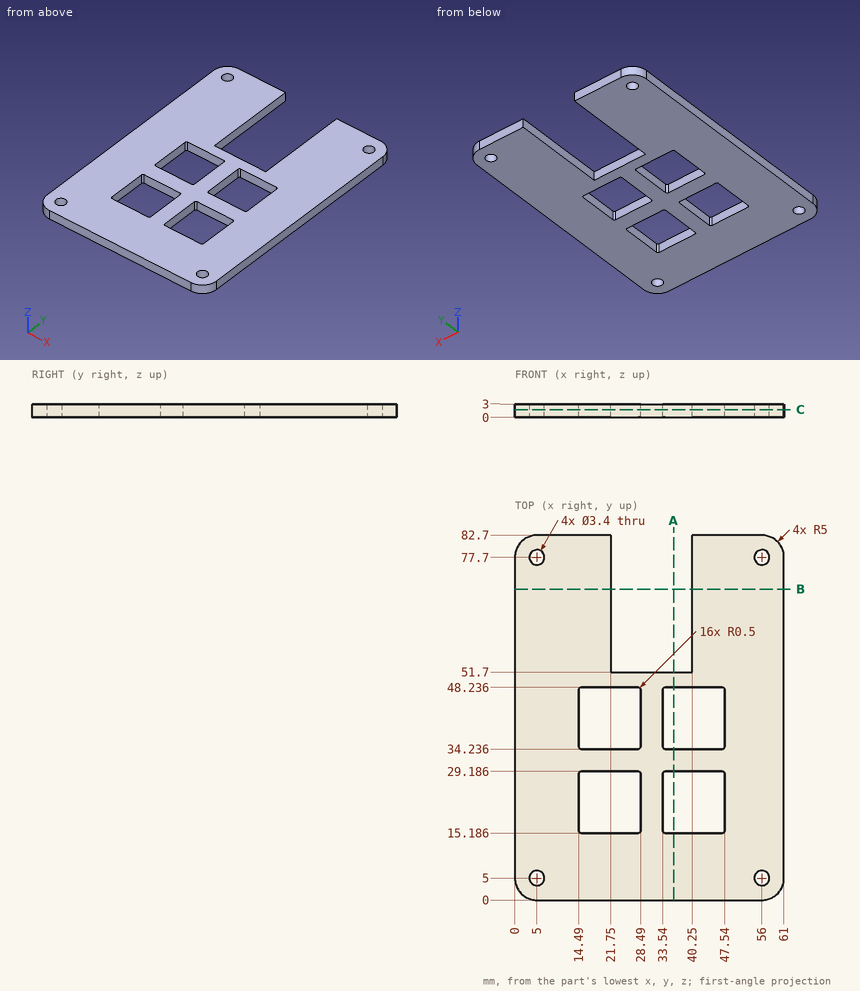
Check sheet for the drawn part. Datum: minimum x, y, z corner. Units: mm. Round coordinates to 2 decimals unless told otherwise and drop trailing zeros. Loops run counter-clockwise (first coordinate to the right, second up) from the corner with the lowest first, then second, coordinate; pieces in that order, holes last. Notation, with made-up numbers: (-37.75, 28.25) - (12.25, 28.25) arc R8 ccw to (12.25, 36.25) - close; hole circle Ø1 at (83.25, -3.75). An arc over 180 degrees is marked (long way). Answer as a JSON object with one key per item and string values. Group by question number.
Q1. Gauge pin test, flat end, axial feed: P1, Ø0.9, axis at x = 28, z = 2, coming from the +Y side. Record the tip position at first contact, or that the pin passes through.
Q2. Sectioned sample at B-B, the plane y = 70.5. Enter the section's corners in (x, z), plus the area to 4 significant figures.
Q3. Sectioned sample at A-A, the plane x = 36. Enter the section's corners in (y, z), plus the area to 3 significant figures.
Q4. Scan lines: line 1 along Y through (x, z) = (27, 0.7); line 2 along Y through (x, z) = (21.5, 1.4); line 3 along X through (y, z) = (42, 2). Record each from-to range of solid material in increasing order. Write a range as [from, to].
Q5. Sectioned sample at C-C, the plane z = 1.75. Count the separate pieces of the cut face and the enclosed holes in it, plus the area to 3 significant figures.
Solution:
{
 "1": {"P1": "stops at y = 51.7"},
 "2": {"outline": "(0, 0) - (21.75, 0) - (21.75, 3) - (0, 3) - close; (40.25, 0) - (61, 0) - (61, 3) - (40.25, 3) - close", "area": "127.5 mm²"},
 "3": {"outline": "(0, 0) - (15.19, 0) - (15.19, 3) - (0, 3) - close; (29.19, 0) - (34.24, 0) - (34.24, 3) - (29.19, 3) - close; (48.24, 0) - (51.7, 0) - (51.7, 3) - (48.24, 3) - close", "area": "71.1 mm²"},
 "4": {"line 1": "y = [0, 15.19], [29.19, 34.24], [48.24, 51.7]", "line 2": "y = [0, 15.19], [29.19, 34.24], [48.24, 82.7]", "line 3": "x = [0, 14.49], [28.49, 33.54], [47.54, 61]"},
 "5": {"separate pieces": "1", "enclosed holes": "8", "area": "3,630 mm²"}
}
